Answer from the drawing. Dimensions are ordinates in mm from the lowest x, y and z of the part. A direction names the side the tool comes from. Round coordinates to 2 decimals unless told otherwise and drop trailing zeros. Write each loop counter-clockwise with the first axis right and the second up, starting at its lowest first coordinate (ties: lowest second). Pieces come first, ordered by that corner, then holes. Notation, with made-up numbers: (-39.5, 20.5) - (-29.5, 20.5) arc R18 cw to (-29.5, 47.5) - close; hole circle Ø9 at (62, -1.75). An arc over 180 degrees is marked (long way). Answer as CSV lines item,"result". Start each with the question number.
1) Consider line 1 along Z through (x, y) = (5, 13); line 2 along X through (y, z) = (14.5, 18); line 3 along Z through (x, y) = (33.5, 2.5). Determine where each line is inside the solid, lowest interval first.
2) Find section C-C on z = 17. Determine the outline of the cut face in (x, y).
3) Find section B-B on x = 17.5. Determine the outline of the cut face in (y, z) (3 decimals).
4) Each of these flat-tipped pins is pushed along its axis until it touches: pin 1 (1 mm diameter, centred on x = 33, z = 15.5, fed in from -Y); pin 2 (3 mm diameter, centred on x = 14.5, z = 15.5, fed in from -Y); pin 3 (10 mm diameter, centred on x = 32.5, y = 23, fed in from +Z); pin 4 (8 mm diameter, centred on y = 7.5, z = 4.5, fed in from -X). Where does it stop, or does it pass through?
5) Which of the six approach directions +Z, -Z, +X, -X, +Y, -Y give full straight-line access (tool end or side, diameter ignored) to the marked faces 1, 2 and 3?
6) Find section D-D on x = 11. Determine the outline of the cut face in (y, z), then the cut area to 3 significant figures.
7) Find section A-A on y = 8. Determine the outline of the cut face in (x, z), then the cut area to 3 significant figures.
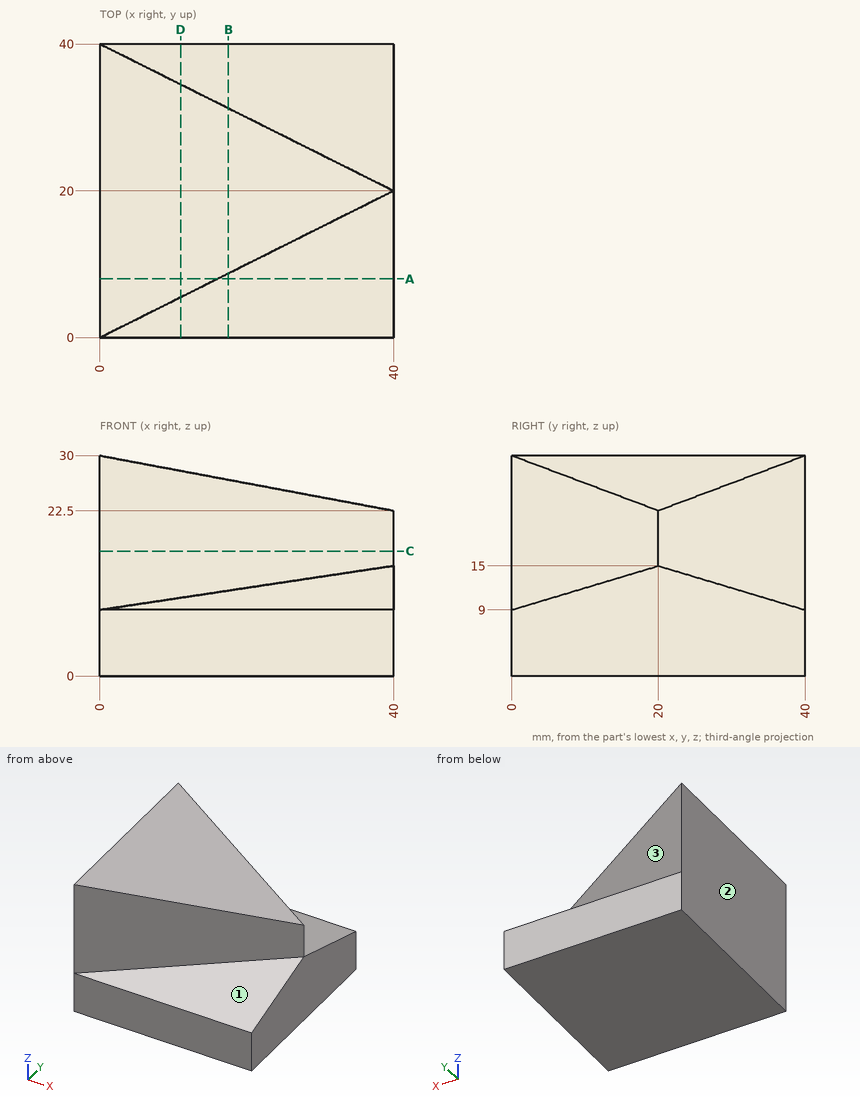
Check values:
1,line 1,"z = 0 to 29.06"
1,line 2,"x = 0 to 29"
1,line 3,"z = 0 to 9.75"
2,outline,"(0, 0) - (40, 20) - (0, 40) - close"
3,outline,"(0, 0) - (40, 0) - (40, 9) - (31.25, 11.625) - (31.25, 26.719) - (8.75, 26.719) - (8.75, 11.625) - (0, 9) - close"
4,pin 1,"stops at y = 16.25"
4,pin 2,"stops at y = 6.5"
4,pin 3,"stops at z = 24.84"
4,pin 4,"stops at x = 0"
5,face 1,"+Z, +X, -Y"
5,face 2,"+Z, -Z, -X, +Y, -Y"
5,face 3,"+Z, +X, +Y"
6,outline,"(0, 0) - (40, 0) - (40, 9) - (34.5, 10.65) - (34.5, 27.94) - (5.5, 27.94) - (5.5, 10.65) - (0, 9) - close"
6,area,"918 mm^2"
7,outline,"(0, 0) - (40, 0) - (40, 11.4) - (16, 11.4) - (16, 27) - (0, 30) - close"
7,area,"730 mm^2"
